For this review, use the dimensioned drawing (mm, ordinates from the lowest corner) and the shaded views. A direction names the side the tool comes from. Coordinates: 2 decimals unless noted, no trailing zeros. Loops run counter-clockwise (first coordinate to the right, second up) from the corner with the lowest first, then second, coordinate; pieces in that order, holes last.
1. To check wall thickness, follow probe 1 along Y at (x, z) = (357, 86.5); probe 2 along Y at (x, z) = (27, 47). State the ranges of each line that lie inside material, in increasing order.
2. Machinability: for the marked faces 4 and 5, which of the approach directions +Z, -Z, +X, -X, +Y, -Y give a long, thin tool a straight path to every point of the face, cutting with its end or side? Answer none if there is none.
3. Take a section at B-B, the plane y = 139.5. State the section outline as (x, z) points.
4. Clearance check with flat-ended pins moving along their axes: P1, Ø3, axis at y = 36.5, z = 122, coming from the +X side; P2, Ø6, axis at x = 112.5, z = 254, coming from the +Y side; P3, Ø22, axis at x = 424, z = 102, coming from the -Y side. State where each tip first meets the part, or that it passes through.
5. Take a section at A-A, the plane z = 187. State the section outline as (x, y) points, then the cut area to 3 significant figures.
6. Mouldability with a two-part tool opening along Y and no side actions: class the marked faces 1, 2 and 3 as pulls with the +Y half, pulls with the -Y half, needs draft (parallel to the pull), parting line crosses it, or undercut.
7. Take a section at C-C, the plane x = 176. State the section outline as (y, z) points.
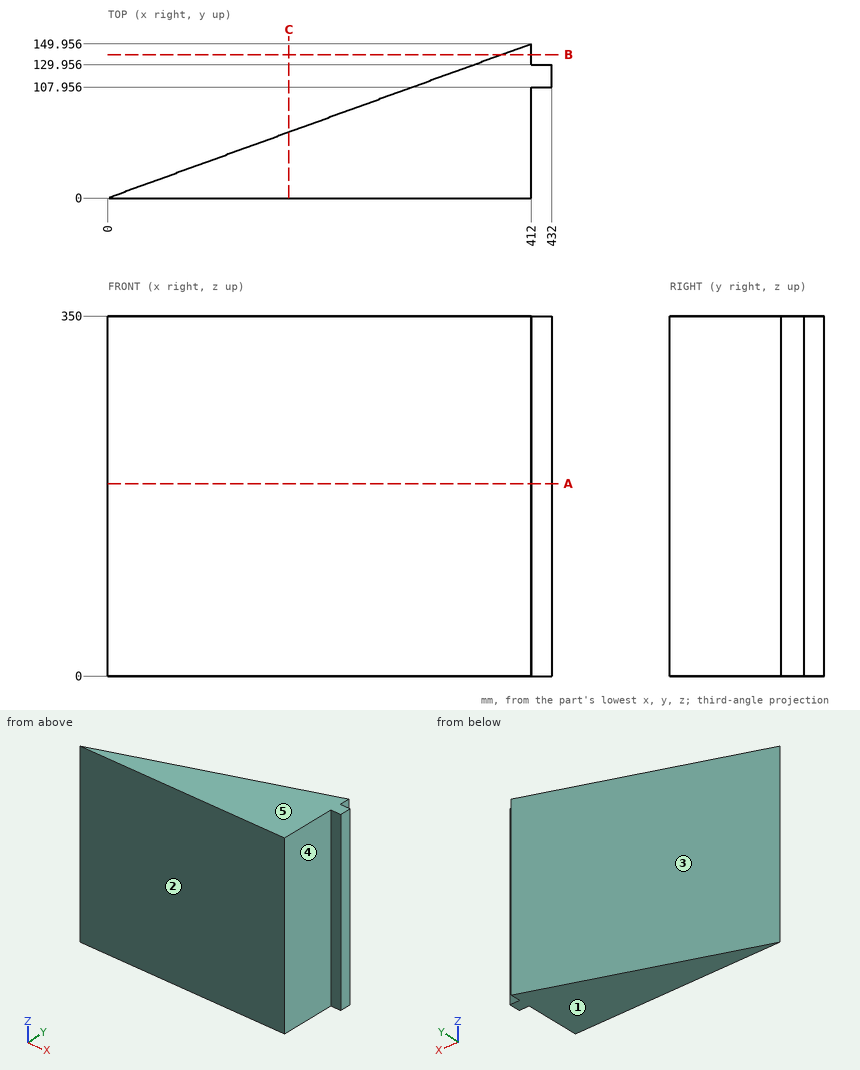
Results list:
1. probe 1: y = 0 to 129.94
1. probe 2: y = 0 to 9.83
2. face 4: +Z, -Z, +X, -Y
2. face 5: +Z, +X, -X, +Y, -Y
3. outline: (383.27, 0) - (412, 0) - (412, 350) - (383.27, 350) - close
4. P1: stops at x = 412
4. P2: stops at y = 42.04
4. P3: stops at y = 107.96
5. outline: (0, 0) - (412, 0) - (412, 107.96) - (432, 107.96) - (432, 129.96) - (412, 129.96) - (412, 149.96) - close
5. area: 31,300 mm2
6. face 1: needs draft
6. face 2: pulls with the -Y half
6. face 3: pulls with the +Y half
7. outline: (0, 0) - (64.06, 0) - (64.06, 350) - (0, 350) - close
